The drawing under review shows one solid part. Ordinate dimensions are in mm from its lowest x, y, z. A direction names the side the tool comes from. Give positions to 0.01 mm unless a question says otherwise; leave off trailing zeros. Order: outer loops, then holes, each group sorted by start corner. A loop starts at its lowest first (then second) coordinate and runs counter-clockwise, first axis right, second up. Notation, with made-up numbers: (25, 5.25) -> (47, 5.25) arc R28 cw to (47, 36.25) -> close; hole circle Ø11 at (-19, 48). An arc over 180 degrees is marked (long way). Use a Markdown table: item, result. Add a question column.
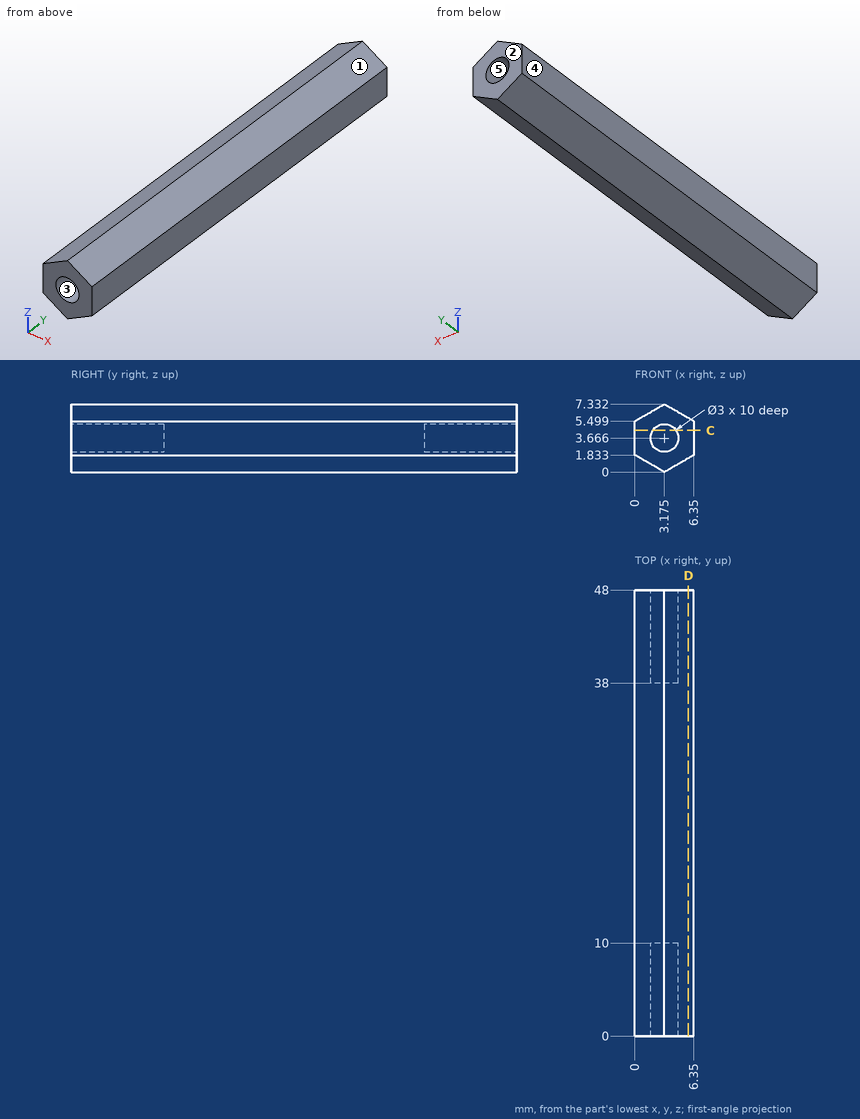
1) For L1, parallel to Y at x = 3, z = 4.5; L2, parallel to Z at x = 4.25, y = 39.5; L3, parallel to Z at x = 5.5, y = 41.5, list the stretches that pass through material, from the lowest coordinate up. Write a range as [from, to].
2) Add section C-C (z = 4.5). Give the boundary of the cut face in (x, y).
3) Insertion check: pin 1 (2 mm diameter, centred on x = 1, y = 36, fed in from -Z); pin 2 (2.5 mm diameter, centred on x = 3.18, z = 3.67, fed in from +Y); pin 3 (1 mm diameter, centred on x = 5, y = 36.5, fed in from -Z) (1 decimal). Each pin has a flat end and moves straight along its axis. Give the tip position at first contact, or say it passes through.
4) Add section D-D (x = 5.75). Give the boundary of the cut face in (y, z) (1 decimal).
5) Machinability: for the marked faces 4 and 5, which of the approach directions +Z, -Z, +X, -X, +Y, -Y give a long, thin tool a straight path to every point of the face, cutting with its end or side? Answer none if there is none.
6) The part is to be moulded in two halves that separate along X. For the marked faces 1, 2 and 3, say which applies: +X half, -X half, draft (parallel to the pull), parting line (faces both ways), or undercut.
Worked answers:
| question | item | result |
|---|---|---|
| 1 | L1 | [10, 38] |
| 1 | L2 | [0.62, 2.62], [4.71, 6.71] |
| 1 | L3 | [1.34, 5.99] |
| 2 | outline | (0, 0) -> (1.93, 0) -> (1.93, 10) -> (4.42, 10) -> (4.42, 0) -> (6.35, 0) -> (6.35, 48) -> (4.42, 48) -> (4.42, 38) -> (1.93, 38) -> (1.93, 48) -> (0, 48) -> close |
| 3 | pin 1 | z = 0.68 |
| 3 | pin 2 | y = 38 |
| 3 | pin 3 | z = 0.8 |
| 4 | outline | (0, 1.5) -> (48, 1.5) -> (48, 5.8) -> (0, 5.8) -> close |
| 5 | face 4 | +Z, -Z, -X, +Y, -Y |
| 5 | face 5 | +Y |
| 6 | face 1 | +X half |
| 6 | face 2 | draft |
| 6 | face 3 | undercut |
